Verification items for the finished model (mm, model axes). Face numbers are marked on the shaded views. A direction names the side the tool comes from. Coordinates: 2 decimals unless noted, no trailing zeros. Write each loop counter-clockwise with the first axis right and the second up, starting at its lowest first coordinate (ties: lowest second). Pieces come first, ordered by that corner, then holes. Notation, with made-up numbers: (20, 14) - (26, 14) arc R30 ccw to (26, 49) - close; hole circle Ø8 at (21, 79.5). An arc over 180 degrees is marked (long way). Use one line per item in the form item = value. Start each with the question number.
(1) Sectioned sample at C-C (y = 3.5). Record the cut outline in (x, z), and give its area (3 significant figures).
(2) Mould release check, pull along Z, two halves, no side actions. Record for the marked faces 1 and 2: released by +Z, released by -Z, zero draft, split by the parting line, or undercut.
(3) Sectioned sample at A-A (x = 0). Record the cut outline in (y, z) (3 decimals), and give its area (3 significant figures).
(4) Tool access check on the marked faces 3 and 4. Record the directions out of +Z, -Z, +X, -X, +Y, -Y that give a thin tool (end or side, any length) a straight path to the whole face; none if there is none.
(5) Material ranges on line 1 (X direction, y = 4, z = 0); line 2 (Y direction, x = -24, z = 8); line 3 (X direction, y = 1.5, z = -5.5), recorded low to high. Write a range as [from, to].
(6) Sectioned sample at B-B (z = 0). Record the cut outline in (x, y) (3 decimals), and give its area (3 significant figures).
(7) Gauge pin test, flat ends, axial feed: pin 1 Ø3 at (y, z) = (6.5, -20) entering from +X; pin 2 Ø2 at (y, z) = (9.5, -9.5) entering from -X; pin 3 Ø5 at (y, z) = (2, -25) entering from +X; pin 4 Ø3 at (x, z) = (25, 26) entering from -Y. Record the tip position at first contact, or that the pin passes through.
from build123d import *

# Parameters (mm, degrees)
IZIM1_R                     = 33
Y_KSEKLIK_EKSTR_ZYON1_DEPTH = 11
IZIM3_R                     = 31
KES_EKSTR_ZYON1_DEPTH       = 7
IZIM4_R                     = 25.925
KES_EKSTR_ZYON2_DEPTH       = 2
RADYUS2_R                   = 1
PAH1_SIZE                   = 5
IZIM5_R                     = 15
KES_EKSTR_ZYON3_DEPTH       = 2


with BuildPart() as part:
    # Çizim1 → Yükseklik-Ekstrüzyon1 (new body)
    with BuildSketch(Plane(origin=(0, 0, 0), x_dir=(1, 0, 0), z_dir=(0, 1, 0))):
        with Locations(Location((0, 0, 0), (0, 0, 270))):
            Circle(IZIM1_R)
    extrude(amount=Y_KSEKLIK_EKSTR_ZYON1_DEPTH)

    # Çizim3 → Kes-Ekstrüzyon1 (cut)
    with BuildSketch(Plane.XZ):
        with Locations(Location((0, 0, 0), (0, 0, 270))):
            Circle(IZIM3_R)
    extrude(amount=-KES_EKSTR_ZYON1_DEPTH, mode=Mode.SUBTRACT)

    # Çizim4 → Kes-Ekstrüzyon2 (cut)
    with BuildSketch(Plane(origin=(0, 11, 0), x_dir=(1, 0, 0), z_dir=(0, 1, 0))):
        with Locations(Location((0, 0, 0), (0, 0, 270))):
            Circle(IZIM4_R)
    extrude(amount=-KES_EKSTR_ZYON2_DEPTH, mode=Mode.SUBTRACT)

    # Radyus2
    radyus2_edges = [part.edges().sort_by_distance(p)[0] for p in [
        (0, 11, -25.925),
    ]]
    fillet(radyus2_edges, radius=RADYUS2_R)

    # Pah1
    pah1_edges = [part.edges().sort_by_distance(p)[0] for p in [
        (0, 11, -33),
    ]]
    chamfer(pah1_edges, length=PAH1_SIZE)

    # Çizim5 → Kes-Ekstrüzyon3 (cut)
    with BuildSketch(Plane(origin=(0, 9, 0), x_dir=(1, 0, 0), z_dir=(0, 1, 0))):
        with Locations(Location((0, 0, 0), (0, 0, 270))):
            Circle(IZIM5_R)
    extrude(amount=-KES_EKSTR_ZYON3_DEPTH, mode=Mode.SUBTRACT)


solid = part.part
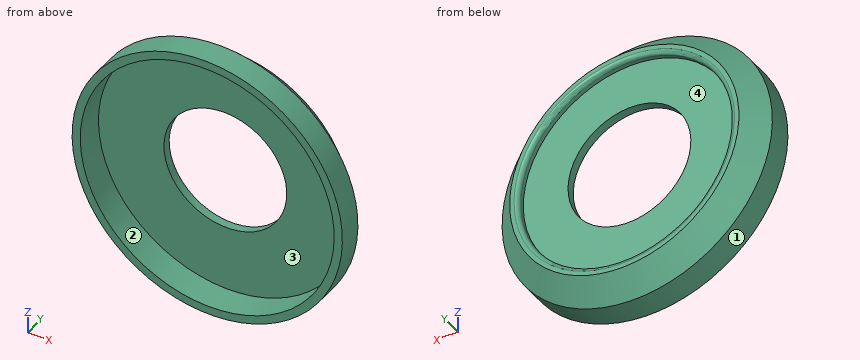
Answers below:
q1.outline = circle Ø66 at (0, 0); hole circle Ø62 at (0, 0)
q1.area = 402 mm2
q2.face_1 = split by the parting line
q2.face_2 = undercut
q3.outline = (0, -33) - (6, -33) - (11, -28) - (11, -26.925) arc R1 ccw to (10, -25.925) - (9, -25.925) - (9, -15) - (7, -15) - (7, -31) - (0, -31) - close; (0, 31) - (7, 31) - (7, 15) - (9, 15) - (9, 25.925) - (10, 25.925) arc R1 ccw to (11, 26.925) - (11, 28) - (6, 33) - (0, 33) - close
q3.area = 103 mm2
q4.face_3 = -Y
q4.face_4 = +Y
q5.line_1 = [-33, -31], [31, 33]
q5.line_2 = [7, 9]
q5.line_3 = [-32.54, -30.51], [30.51, 32.54]
q6.outline = (-33, 0) - (-31, 0) - (-31, 7) - (-15, 7) - (-15, 9) - (-25.925, 9) - (-25.925, 10) arc R1 ccw to (-26.925, 11) - (-28, 11) - (-33, 6) - close; (15, 7) - (31, 7) - (31, 0) - (33, 0) - (33, 6) - (28, 11) - (26.925, 11) arc R1 ccw to (25.925, 10) - (25.925, 9) - (15, 9) - close
q6.area = 103 mm2
q7.pin_1 = 27.27
q7.pin_2 = -29.03
q7.pin_3 = 24.14
q7.pin_4 = through
